Part model, mm, in its own coordinate system. Face numbers are marked on the shaded views. A direction names the side the tool comes from. Coordinates: 2 decimals unless noted, no trailing zeros. Write each loop counter-clockwise with the first axis right and the second up, starting at its lowest first coordinate (ties: lowest second). Pieces come first, ordered by that corner, then holes. Notation, with made-up numbers: (25.5, 9.25) - (70.5, 9.25) arc R20 ccw to (70.5, 36.25) - close; hole circle Ø5 at (50, 24.5). An arc over 180 degrees is marked (long way). Use a Markdown table: item, result.
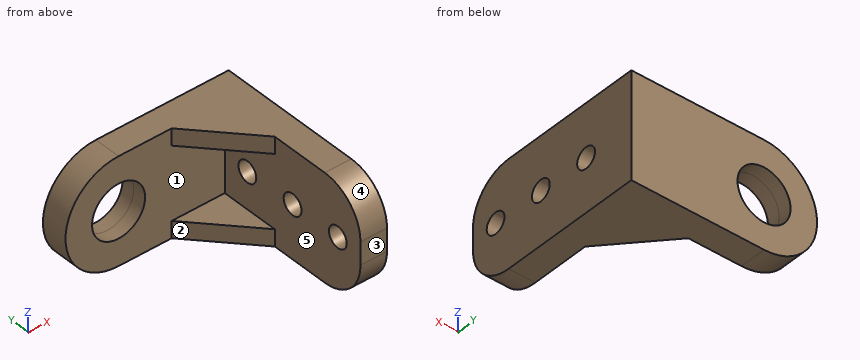
```python
from build123d import *

# Parameters (mm, degrees)
SKETCH1_R           = 12.7
SKETCH1_R_2         = 6.35
BOSS_EXTRUDE1_DEPTH = 3.175
SKETCH2_W           = 6.35
SKETCH2_H           = 38.1
BOSS_EXTRUDE2_DEPTH = 25.4
SKETCH3_R           = 2.5
CUT_EXTRUDE1_DEPTH  = 58.589283942
FILLET1_R           = 10
RIB13_REACH         = 58.3
SKETCH4_WALL_W      = 133.538435182
SKETCH4_WALL_H      = 4


with BuildPart() as part:
    # Sketch1 → Boss-Extrude1 (new, symmetric)
    # profile 1 of 3: a face of its own
    with BuildSketch(Plane(origin=(0, 0, 0), x_dir=(1, 0, 0), z_dir=(0, 1, 0))):
        Circle(SKETCH1_R)
        with Locations(Location((0, 0, 0), (0, 0, 270))):
            Circle(SKETCH1_R_2, mode=Mode.SUBTRACT)
    # profile 2 of 3: a face of its own
    with BuildSketch(Plane(origin=(0, 0, 0), x_dir=(1, 0, 0), z_dir=(0, 1, 0))):
        with BuildLine():
            Line((31.75, 12.7), (12.7, 12.7))
            Line((12.7, 12.7), (12.7, 0))
            ThreePointArc((12.7, 0), (8.980256121, -8.980256121), (0, -12.7))
            Line((0, -12.7), (31.75, -12.7))
            Line((31.75, -12.7), (31.75, 12.7))
        make_face()
    # profile 3 of 3: a face of its own
    with BuildSketch(Plane(origin=(0, 0, 0), x_dir=(1, 0, 0), z_dir=(0, 1, 0))):
        with BuildLine():
            Line((12.7, 12.7), (0, 12.7))
            ThreePointArc((0, 12.7), (8.980256121, 8.980256121), (12.7, 0))
            Line((12.7, 0), (12.7, 12.7))
        make_face()
    extrude(amount=BOSS_EXTRUDE1_DEPTH, both=True)

    # Sketch2 → Boss-Extrude2 (add)
    with BuildSketch(Plane.XY.offset(12.7)):
        with Locations((28.575, -22.225)):
            Rectangle(SKETCH2_W, SKETCH2_H)
    extrude(amount=-BOSS_EXTRUDE2_DEPTH)

    # Sketch3 → Cut-Extrude1 (cut, through all)
    with BuildSketch(Plane.ZY.offset(-25.4)):
        with Locations(Location((0, -34.925, 0), (0, 0, 270))):
            Circle(SKETCH3_R)
        with Locations(Location((0, -9.525, 0), (0, 0, 270))):
            Circle(SKETCH3_R)
        with Locations(Location((0, -22.225, 0), (0, 0, 270))):
            Circle(SKETCH3_R)
    extrude(amount=-CUT_EXTRUDE1_DEPTH, mode=Mode.SUBTRACT)

    # Fillet1
    fillet1_edges = [part.edges().sort_by_distance(p)[0] for p in [
        (28.575, -41.275, 12.7),
        (28.575, -41.275, -12.7),
    ]]
    fillet(fillet1_edges, radius=FILLET1_R)

    # Sketch4 wall → Rib13 (add, up to next)
    with BuildSketch(Plane(origin=(19.05, -10.2, 8.7), x_dir=(0.670567611254, -0.741848420324, 0), z_dir=(0.741848420324, 0.670567611254, 0)), mode=Mode.PRIVATE) as rib13_sk1:
        with Locations((0, -2)):
            Rectangle(SKETCH4_WALL_W, SKETCH4_WALL_H)
    rib13_tool1 = extrude(rib13_sk1.sketch, amount=RIB13_REACH, mode=Mode.PRIVATE) - part.part
    rib13 = rib13_tool1.solids().sort_by_distance((19.05, -10.2, 8.7))[0]
    add(rib13)

    # Mirror1: Rib13 across plane
    add(rib13.mirror(Plane.XY))


solid = part.part
```
Item 1: Band-saw the part on B-B, the plane y = -1. Give the cut face in (x, z).
From the geometry:
| item | result |
|---|---|
| outline | (0, -12.7) - (31.75, -12.7) - (31.75, 12.7) - (0, 12.7) arc R12.7 ccw to start; hole circle Ø12.7 at (0, 0) |
Item 2: Band-saw the part on A-A, the plane z = 0. Give the cut face in (x, y) (3 decimals), then the cut area to 3 significant figures.
From the geometry:
| item | result |
|---|---|
| outline | (-12.7, -3.175) - (-6.35, -3.175) - (-6.35, 3.175) - (-12.7, 3.175) - close; (6.35, -3.175) - (25.4, -3.175) - (25.4, -7.025) - (31.75, -7.025) - (31.75, 3.175) - (6.35, 3.175) - close; (25.4, -41.275) - (31.75, -41.275) - (31.75, -37.425) - (25.4, -37.425) - close; (25.4, -32.425) - (31.75, -32.425) - (31.75, -24.725) - (25.4, -24.725) - close; (25.4, -19.725) - (31.75, -19.725) - (31.75, -12.025) - (25.4, -12.025) - close |
| area | 348 mm^2 |
Item 3: Band-saw the part on C-C, the plane x = -5.5. Give the cut face in (y, z) (3 decimals), then the cut area to 3 significant figures.
From the geometry:
| item | result |
|---|---|
| outline | (-3.175, -11.447) - (3.175, -11.447) - (3.175, -3.174) - (-3.175, -3.174) - close; (-3.175, 3.174) - (3.175, 3.174) - (3.175, 11.447) - (-3.175, 11.447) - close |
| area | 105 mm^2 |
Item 4: Drop flat-ended pins along their axis: P1, Ø12.5, axis at y = -22.5, z = 2, coming from the -X side; P2, Ø5, axis at x = 17, y = -10.5, coming from the -Z side; P3, Ø12.5, axis at x = 0.5, z = 1.5, coming from the -Y side (3 decimals). Give the stop position or say it passes through.
From the geometry:
| item | result |
|---|---|
| P1 | x = 25.4 |
| P2 | z = -12.7 |
| P3 | y = -3.175 |
Item 5: Drill centre lines: probe 1 along Z at (x, y) = (24, -3.5); probe 2 along X at (y, z) = (-7, -8); probe 3 along Y at (x, z) = (-3.5, -5.75) (3 decimals). Where is each one in solid material? Low to high.
From the geometry:
| item | result |
|---|---|
| probe 1 | -12.7 to -8.7, 8.7 to 12.7 |
| probe 2 | 25.4 to 31.75 |
| probe 3 | -3.175 to 3.175 |
Item 6: Two-plate mould, pull along Z, no slides. Class the marked faces 3, 4 and 5: pulls with the +Z half, pulls with the -Z half, needs draft (parallel to the pull), parting line crosses it, or undercut.
From the geometry:
| item | result |
|---|---|
| face 3 | needs draft |
| face 4 | pulls with the +Z half |
| face 5 | undercut |
Item 7: Band-saw the part on D-D, the plane y = -35.5. Give the cut face in (x, z), then the cut area to 3 significant figures.
From the geometry:
| item | result |
|---|---|
| outline | (25.4, -11.76) - (31.75, -11.76) - (31.75, -2.43) - (25.4, -2.43) - close; (25.4, 2.43) - (31.75, 2.43) - (31.75, 11.76) - (25.4, 11.76) - close |
| area | 118 mm^2 |
Item 8: Which spindle directions (+Z, -Z, +X, -X, +Y, -Y) get a long thin tool onto all of the face, cutting with end or side? Do the marked faces 1 and 2. Say none if no direction does.
From the geometry:
| item | result |
|---|---|
| face 1 | -X, -Y |
| face 2 | +Z, -Z, -X, -Y |
